from build123d import *

# Parameters (mm, degrees)
F1_DEPTH = 3.048
F2_R     = 2.38125
F3_DEPTH = 3.048
F4_R     = 3.571875
F5_DEPTH = 9.525
F6_R     = 2.38125
F7_DEPTH = 6.35


with BuildPart() as f1:
    # F0 (on Top) → F1 (new body)
    with BuildSketch(Plane.XY):
        with BuildLine():
            Line((356.6070268588, 293.1853402508), (89.9070268588, 293.1853402508))
            Line((89.9070268588, 293.1853402508), (89.9070268588, 230.838141456))
            ThreePointArc((89.9070268588, 230.838141456), (88.5285448509, 226.3678853975), (84.8718925649, 223.4503014769))
            Line((84.8718925649, 223.4503014769), (25.6127064183, 200.1699069193))
            ThreePointArc((25.6127064183, 200.1699069193), (24.3322333387, 199.4889237751), (23.2396710643, 198.5351643577))
            ThreePointArc((23.2396710643, 198.5351643577), (-1.2970857024, 134.0019257775), (24.7815527961, 70.0762194589))
            Line((24.7815527961, 70.0762194589), (99.2751600757, -4.4173878207))
            ThreePointArc((99.2751600757, -4.4173878207), (105.4554248707, -8.5469087335), (112.7455442573, -9.9970036391))
            Line((112.7455442573, -9.9970036391), (373.8109154673, -9.9970036391))
            ThreePointArc((373.8109154673, -9.9970036391), (385.6186847653, -5.8962204817), (392.3428738571, 4.6406253157))
            Line((392.3428738571, 4.6406253157), (420.6077241059, 123.3529963609))
            ThreePointArc((420.6077241059, 123.3529963609), (416.1467307829, 211.7798908878), (356.6070268588, 277.3103402508))
            Line((356.6070268588, 277.3103402508), (356.6070268588, 293.1853402508))
        make_face()
    extrude(amount=F1_DEPTH)

    # F2 (on face) → F3 (cut, through all)
    with BuildSketch(Plane.XY.offset(3.048)):
        with Locations((261.3570268588, 283.6603402508)):
            Circle(F2_R)
        with Locations((197.8570268588, 283.6603402508)):
            Circle(F2_R)
        with Locations((134.3570268588, 283.6603402508)):
            Circle(F2_R)
    extrude(amount=-F3_DEPTH, mode=Mode.SUBTRACT)

    # F4 (on face) → F5 (cut)
    with BuildSketch(Plane.XY.offset(3.048)):
        with Locations((99.4320268588, 181.6634652508)):
            Circle(F4_R)
        with Locations((16.8820268588, 140.7853402508)):
            Circle(F4_R)
        with Locations((305.8070268588, 194.7603402508)):
            Circle(F4_R)
    extrude(amount=-F5_DEPTH, mode=Mode.SUBTRACT)

    # F6 (on face) → F7 (cut)
    with BuildSketch(Plane.XY.offset(3.048)):
        with BuildLine():
            Line((44.1701730803, 207.4603402508), (417.85350826, 207.4603402508))
            ThreePointArc((417.85350826, 207.4603402508), (393.6078526777, 247.9773896185), (356.6070268588, 277.3103402508))
            Line((356.6070268588, 277.3103402508), (356.6070268588, 293.1853402508))
            Line((356.6070268588, 293.1853402508), (89.9070268588, 293.1853402508))
            Line((89.9070268588, 293.1853402508), (89.9070268588, 230.838141456))
            ThreePointArc((89.9070268588, 230.838141456), (88.5285448509, 226.3678853975), (84.8718925649, 223.4503014769))
            Line((84.8718925649, 223.4503014769), (44.1701730803, 207.4603402508))
        make_face()
        with Locations((134.3570268588, 283.6603402508)):
            Circle(F6_R, mode=Mode.SUBTRACT)
        with Locations((197.8570268588, 283.6603402508)):
            Circle(F6_R, mode=Mode.SUBTRACT)
        with Locations((261.3570268588, 283.6603402508)):
            Circle(F6_R, mode=Mode.SUBTRACT)
    extrude(amount=-F7_DEPTH, mode=Mode.SUBTRACT)


solid = f1.part
Design review of the part built by this model. Coordinates are the model's own, in mm. Round coordinates to 2 decimals unless told otherwise and drop trailing zeros. Order: outer loops, then holes, each group sorted by start corner. A loop starts at its lowest first (then second) coordinate and runs counter-clockwise, first axis right, second up. Notation, with made-up numbers: M 83.5,44 L 94.5,44 A31 cw 94.5,77 Z; hole C 62,-24.75 d3. An arc over 180 degrees is marked long. Answer as CSV lines item,"result". Start each with the question number.
1) Wall thickness on line 1 along X through (y, z) = (197, 1.6); line 2 along X through (y, z) = (19, 1.05); line 3 along X through (y, z) = (157.5, 2.7): over which ranges is each line inside the solid? List them lowest first. Write a range as [from, to].
2) Add section C-C (x = 87). Give the boundary of the cut face in (y, z).
3) Add section A-A (z = 1.1). Give the boundary of the cut face in (x, y), then the cut area to 3 significant figures.
4) Add section B-B (y = 21.5). Give the boundary of the cut face in (x, z), then the cut area to 4 significant figures.
Resolved:
1,line 1,"[21.87, 303.02], [308.59, 421.28]"
1,line 2,"[75.86, 395.76]"
1,line 3,"[1.39, 426.16]"
2,outline,"M 7.86,0 L 207.46,0 L 207.46,3.05 L 7.86,3.05 Z"
3,outline,"M 23.24,198.54 A94.17 ccw 24.78,70.08 L 99.28,-4.42 A19.05 ccw 112.75,-10 L 373.81,-10 A19.05 ccw 392.34,4.64 L 420.61,123.35 A131.42 ccw 417.85,207.46 L 44.17,207.46 L 25.61,200.17 A6.35 ccw Z; hole C 16.88,140.79 d7.14; hole C 99.43,181.66 d7.14; hole C 305.81,194.76 d7.14"
3,area,"83,100 mm^2"
4,outline,"M 73.36,0 L 396.36,0 L 396.36,3.05 L 73.36,3.05 Z"
4,area,"984.5 mm^2"
